The model under review builds one solid part; all positions refer to its coordinate system, in mm. A direction names the side the tool comes from. Give positions to 0.01 mm unless a question says otherwise; leave off trailing zeros. Order: outer loops, then holes, each group sorted by start corner. A loop starts at its lowest first (then second) coordinate and runs counter-clockwise, first axis right, second up.
```python
from build123d import *

# Parameters (mm, degrees)
F0_W     = 350
F0_H     = 350
F1_DEPTH = 10
F2_W     = 320
F2_H     = 320
F3_DEPTH = 8
F4_R     = 2.5


with BuildPart() as f1:
    # F0 (on Top) → F1 (new body)
    with BuildSketch(Plane.XY):
        Rectangle(F0_W, F0_H)
    extrude(amount=F1_DEPTH)

    # F2 (on face) → F3 (cut)
    with BuildSketch(Plane.XY.offset(10)):
        Rectangle(F2_W, F2_H)
    extrude(amount=-F3_DEPTH, mode=Mode.SUBTRACT)

    # F4
    f4_edges = [f1.edges().sort_by_distance(p)[0] for p in [
        (175, -175, 5),
        (175, 0, 10),
        (0, -175, 10),
        (-175, -175, 5),
        (-175, 0, 10),
        (0, 175, 10),
        (-175, 175, 5),
        (175, 175, 5),
    ]]
    fillet(f4_edges, radius=F4_R)


solid = f1.part
```
Item 1: Clearance check with a flat-ended pin moving along its axis: pin 1 Ø5 at (x, y) = (-17, 97.5) entering from +Z. State where the tip first meets the part, or that it passes through.
Values found:
pin 1: stops at z = 2
Item 2: For line 1 (Y direction, x = 82, z = 3.75); line 2 (X direction, y = -148, z = 8), list the stretches that pass through material, from the lowest coordinate up.
Values found:
line 1: y = -175 to -160, 160 to 175
line 2: x = -174.95 to -160, 160 to 174.95
Item 3: For faces 4 (the flat face through (175, -2, 4)), 5 (the flat face through (-2, 2, 2)), list the 3-axis set-ups (+Z, -Z, +X, -X, +Y, -Y) from which the entire face can be reached by the end or side of a thin tool; tool diameter is ignored.
Values found:
face 4: +Z, -Z, +X, +Y, -Y
face 5: +Z
Item 4: Take a section at A-A (z = 3.75). Give the boundary of the cut face in (x, y).
Values found:
outline: (-175, -172.5) arc R2.5 ccw to (-172.5, -175) - (172.5, -175) arc R2.5 ccw to (175, -172.5) - (175, 172.5) arc R2.5 ccw to (172.5, 175) - (-172.5, 175) arc R2.5 ccw to (-175, 172.5) - close; hole (-160, -160) - (160, -160) - (160, 160) - (-160, 160) - close
Item 5: Draft analysis for pull direction Y (two halves, no side actions). For faces 1 (the flat face through (-160, -2, 6)), 2 (the flat face through (-2, 175, 4)), 3 (the flat face through (-14, -165, 10)), state which applies: released by +Y, released by -Y, zero draft, split by the parting line, or undercut.
Values found:
face 1: undercut
face 2: released by +Y
face 3: zero draft
Item 6: Take a section at B-B (y = -34). Give the boundary of the cut face in (x, z), and give its area (3 significant figures).
Values found:
outline: (-175, 0) - (175, 0) - (175, 7.5) arc R2.5 ccw to (172.5, 10) - (160, 10) - (160, 2) - (-160, 2) - (-160, 10) - (-172.5, 10) arc R2.5 ccw to (-175, 7.5) - close
area: 937 mm2
